Read the model definition and answer for the solid it produces. Units are mm, in the model's axes. A direction names the side the tool comes from. Coordinates: 2 decimals unless noted, no trailing zeros. Write each loop counter-clockwise with the first axis right and the second up, starting at its lowest first coordinate (ties: lowest second). Pieces come first, ordered by that corner, then holes. Notation, with made-up numbers: M -2,61.25 L 14,61.25 A20 cw 14,80.25 Z; hole C 46,-9.75 d2. An arc over 180 degrees is marked long. Write item = value, one per line.
from build123d import *

# Parameters (mm, degrees)
SKIZZE1_R                       = 13
AUFSATZ_LINEAR_AUSTRAGEN1_DEPTH = 20
AUFSATZ_LINEAR_START            = 4
SKIZZE5_R                       = 25
AUFSATZ_LINEAR_AUSTRAGEN2_DEPTH = 4
DURCHGANGSLOCH_F_R_M51_D        = 5.5
DURCHGANGSLOCH_F_R_M51_DEPTH    = 25
DURCHGANGSLOCH_F_R_M51_TIP      = 1.652366702
FASE1_SIZE                      = 1


with BuildPart() as part:
    # Skizze1 → Aufsatz-Linear austragen1 (new body)
    with BuildSketch(Plane(origin=(0, 0, 0), x_dir=(1, 0, 0), z_dir=(0, 1, 0))):
        with Locations(Location((0, 0, 0), (0, 0, 270))):
            Circle(SKIZZE1_R)
        with BuildLine():
            Line((-4.472135955, 4), (4.472135955, 4))
            ThreePointArc((4.472135955, 4), (6, 0), (4.472135955, -4))
            Line((4.472135955, -4), (-4.472135955, -4))
            ThreePointArc((-4.472135955, -4), (-6, 0), (-4.472135955, 4))
        make_face(mode=Mode.SUBTRACT)
    extrude(amount=AUFSATZ_LINEAR_AUSTRAGEN1_DEPTH)

    # Skizze5 → Aufsatz-Linear austragen2 (add)
    with BuildSketch(Plane.XZ.offset(AUFSATZ_LINEAR_START)):
        with Locations(Location((0, 0, 0), (0, 0, 270))):
            Circle(SKIZZE5_R)
        with BuildLine():
            Line((4.472135955, -4), (-4.472135955, -4))
            ThreePointArc((-4.472135955, -4), (-6, 0), (-4.472135955, 4))
            Line((-4.472135955, 4), (4.472135955, 4))
            ThreePointArc((4.472135955, 4), (6, 0), (4.472135955, -4))
        make_face(mode=Mode.SUBTRACT)
    extrude(amount=-AUFSATZ_LINEAR_AUSTRAGEN2_DEPTH)

    # Durchgangsloch für M51
    with Locations(Plane(origin=(0, -4, 0), x_dir=(-1, 0, 0), z_dir=(0, -1, 0))):
        with Locations((0, 20), (20, 0), (0, -20), (-20, 0)):
            Hole(DURCHGANGSLOCH_F_R_M51_D / 2, depth=DURCHGANGSLOCH_F_R_M51_DEPTH)
            with Locations((0, 0, -(DURCHGANGSLOCH_F_R_M51_DEPTH + DURCHGANGSLOCH_F_R_M51_TIP / 2))):  # 118° drill point
                Cone(0, DURCHGANGSLOCH_F_R_M51_D / 2, DURCHGANGSLOCH_F_R_M51_TIP, mode=Mode.SUBTRACT)

    # Fase1
    fase1_edges = [part.edges().sort_by_distance(p)[0] for p in [
        (0, 0, 25),
        (0, 20, -13),
    ]]
    chamfer(fase1_edges, length=FASE1_SIZE)


solid = part.part
Item 1: Find section C-C (y = 15). Determine the outline of the cut face in (x, z), and give its area (3 significant figures).
Worked answers:
outline = C 0,0 d26; hole M -4.47,-4 L 4.47,-4 A6 ccw 4.47,4 L -4.47,4 A6 ccw Z
area = 443 mm²
Item 2: For a pull along X with two mould halves and no side action, classify faces 1 (the face through (-22.747, -1.972, -0.121)), 2 (the face through (-10, 0, -10)), 3 (the face through (7.509, -2.521, -23.846)) as released by +X, released by -X, zero draft, split by the parting line, or undercut.
Worked answers:
face_1 = undercut
face_2 = zero draft
face_3 = split by the parting line
Item 3: Consider line 1 along Y through (x, z) = (17.5, -2); line 2 along X through (y, z) = (-2.9, -20); line 3 along Z through (x, y) = (-3, 10.75). Determine where each line is inside the solid, lowest interval first. Write a range as from..to.
Worked answers:
line_1 = -4..0
line_2 = -15..-2.75, 2.75..15
line_3 = -12.65..-4, 4..12.65
Item 4: Find section B-B (z = 0). Determine the outline of the cut face in (x, y).
Worked answers:
outline = M -25,-4 L -22.75,-4 L -22.75,0 L -24,0 L -25,-1 Z; M -17.25,-4 L -6,-4 L -6,20 L -12,20 L -13,19 L -13,0 L -17.25,0 Z; M 6,-4 L 17.25,-4 L 17.25,0 L 13,0 L 13,19 L 12,20 L 6,20 Z; M 22.75,-4 L 25,-4 L 25,-1 L 24,0 L 22.75,0 Z
Item 5: Find section A-A (x = 0). Determine the outline of the cut face in (y, z), and give its area (3 significant figures).
Worked answers:
outline = M -4,-25 L -1,-25 L 0,-24 L 0,-22.75 L -4,-22.75 Z; M -4,-17.25 L 0,-17.25 L 0,-13 L 19,-13 L 20,-12 L 20,-4 L -4,-4 Z; M -4,4 L 20,4 L 20,12 L 19,13 L 0,13 L 0,17.25 L -4,17.25 Z; M -4,22.75 L 0,22.75 L 0,24 L -1,25 L -4,25 Z
area = 482 mm²
Item 6: Which of the six approach directions +Z, -Z, +X, -X, +Y, -Y give full straight-line access (tool end or side, diameter ignored) to faces 4 (the face through (0, 20, 5)), 5 (the face through (6, 8, 0)), 6 (the face through (-7.91, 9.367, -10.316))?
Worked answers:
face_4 = +Z, -Z, +X, -X, +Y
face_5 = +Y, -Y
face_6 = +Y
Item 7: Flat-ended cylindrical pins translate along their axes: pin 1 (4.5 mm diameter, centred on x = 2, y = 12.5, fed in from -Z); pin 2 (6.5 mm diameter, centred on x = 0, z = 20, fed in from +Y); pin 3 (6 mm diameter, centred on x = 8, y = 8.5, fed in from -Z). Find the tip coordinate at first contact, or state that the pin passes through.
Worked answers:
pin_1 = -13
pin_2 = 0
pin_3 = -12
